Build history of the part. All positions in model axes, mm. A direction names the side the tool comes from. Coordinates: 2 decimals unless noted, no trailing zeros. Order: outer loops, then holes, each group sorted by start corner. A loop starts at its lowest first (then second) coordinate and runs counter-clockwise, first axis right, second up. Notation, with made-up numbers: (-5.75, -10) - (25.25, -10) arc R35 ccw to (25.25, 26) - close; hole circle Ø11 at (-28.5, 45.25). An arc over 180 degrees is marked (long way). Write each question's results on one line, items separated by ' | '.
from build123d import *

# Parameters (mm, degrees)
BOX011_W     = 11.5
BOX011_H     = 49
BOX011_DEPTH = 8
BOX010_W     = 22
BOX010_H     = 49
BOX010_DEPTH = 3.3
FILLET006_R  = 1
BOX012_W     = 15
BOX012_H     = 49
BOX012_DEPTH = 3


with BuildPart() as box011:
    # Box011 → Box011 (new body)
    with BuildSketch(Plane(origin=(-38, -0.2, 84.5), x_dir=(1, 0, 0), z_dir=(0, 0, 1))):
        with Locations((5.75, 24.5)):
            Rectangle(BOX011_W, BOX011_H)
    extrude(amount=BOX011_DEPTH)


with BuildPart() as fillet006:
    # Box010 → Box010 (new body)
    with BuildSketch(Plane(origin=(-43, -0.2, 84.5), x_dir=(1, 0, 0), z_dir=(0, 0, 1))):
        with Locations((11, 24.5)):
            Rectangle(BOX010_W, BOX010_H)
    extrude(amount=BOX010_DEPTH)

    # Fillet006
    fillet006_edges = [fillet006.edges().sort_by_distance(p)[0] for p in [
        (-43, -0.2, 86.15),
        (-43, 48.8, 86.15),
        (-21, -0.2, 86.15),
        (-21, 48.8, 86.15),
    ]]
    fillet(fillet006_edges, radius=FILLET006_R)


with BuildPart() as fusion002007:
    # Box012 → Box012 (new body)
    with BuildSketch(Plane(origin=(-39.5, -0.2, 82), x_dir=(1, 0, 0), z_dir=(0, 0, 1))):
        with Locations((7.5, 24.5)):
            Rectangle(BOX012_W, BOX012_H)
    extrude(amount=BOX012_DEPTH)

    # Fusion002007: union Box011, Fillet006
    add(box011.part)
    add(fillet006.part)


with BuildPart() as fusion002007_1:
    # Fusion002007 placement: moved
    add(fusion002007.part.moved(Location((0, 0, -42))))


solid = fusion002007_1.part
1. Probe line 1 (X direction, y = 3, z = 47); line 2 (X direction, y = 27.5, z = 41); line 3 (Z direction, x = -24, y = 47.5). List the from-to ranges inside material, lowest first.
Solved:
line 1: x = -38 to -26.5 | line 2: x = -39.5 to -24.5 | line 3: z = 42.5 to 45.8
2. Band-saw the part on A-A on y = 45. Give the cut face in (x, z), then the cut area to 3 significant figures.
Solved:
outline: (-43, 42.5) - (-39.5, 42.5) - (-39.5, 40) - (-24.5, 40) - (-24.5, 42.5) - (-21, 42.5) - (-21, 45.8) - (-26.5, 45.8) - (-26.5, 50.5) - (-38, 50.5) - (-38, 45.8) - (-43, 45.8) - close | area: 164 mm2
3. Drop flat-ended pins along their axis: pin 1 Ø4 at (y, z) = (31, 49) entering from -X; pin 2 Ø5 at (y, z) = (33, 48.5) entering from +X; pin 3 Ø1.2 at (y, z) = (27.5, 41.5) entering from +X. Give the stop position or say it passes through.
Solved:
pin 1: stops at x = -38 | pin 2: stops at x = -26.5 | pin 3: stops at x = -24.5
4. Tool access for faces 1 (the face through (-42.715, 48.499, 44.173)), 2 (the face through (-24, 25, 45.8)), 3 (the face through (-24.5, 24, 41)), 4 (the face through (-39.5, 24, 41)), 5 (the face through (-41, 25, 45.8)): list every direction of +Z, -Z, +X, -X, +Y, -Y with a clear straight run to the whole face (end or side of a thin tool).
Solved:
face 1: +Z, -Z, -X, +Y | face 2: +Z, +X, +Y, -Y | face 3: -Z, +X, +Y, -Y | face 4: -Z, -X, +Y, -Y | face 5: +Z, -X, +Y, -Y
5. Band-saw the part on C-C on z = 41.25. Give the cut face in (x, y).
Solved:
outline: (-39.5, -0.2) - (-24.5, -0.2) - (-24.5, 48.8) - (-39.5, 48.8) - close
6. Band-saw the part on B-B on x = -38.5. Give the cut face in (y, z).
Solved:
outline: (-0.2, 40) - (48.8, 40) - (48.8, 45.8) - (-0.2, 45.8) - close
